Check sheet for the modelled part. Datum: model origin and axes. Units: mm. Face numbers are marked on the shaded views. A direction names the side the tool comes from. Coordinates: 2 decimals unless noted, no trailing zeros. Order: outer loops, then holes, each group sorted by start corner. A loop starts at its lowest first (then second) coordinate and runs counter-clockwise, first axis right, second up.
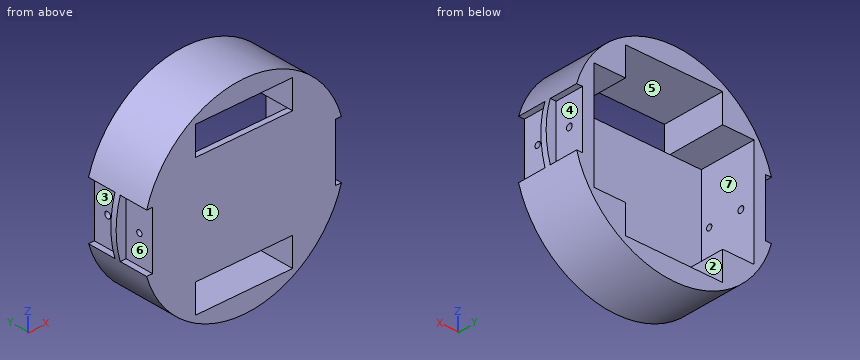
Autodesk Inventor part; units mm, degrees
ref_plane "YZ Plane" through (0, 0, 0) normal (1, 0, 0) x (0, 1, 0)
ref_plane "XZ Plane" through (0, 0, 0) normal (0, 1, 0) x (-1, 0, 0)
ref_plane "XY Plane" through (0, 0, 0) normal (0, 0, 1) x (1, 0, 0)
sketch "Szkic1" plane through (0, 0, 0) normal (0, 1, 0) x (-1, 0, 0)
  circle A0 centre (0, 0) radius 35.5
  line L0 (0, 18.75) -> (0, -18.75) construction
  line L1 (-28, 0) -> (28, 0) construction
  line L2 (-28, -18.75) -> (28, -18.75)
  line L3 (-28, 18.75) -> (-28, -18.75)
  line L4 (28, 18.75) -> (28, -18.75)
  line L5 (0, 18.75) -> (28, 18.75)
  line L6 (0, 18.75) -> (-28, 18.75)
  line L7 (0, 18.75) -> (0, 28.75) construction
  line L8 (17, 28.75) -> (-17, 28.75)
  line L9 (17, 28.75) -> (17, 18.75)
  line L10 (-17, 28.75) -> (-17, 18.75)
  line L11 (0, -18.75) -> (0, -28.75) construction
  line L12 (-17, -28.75) -> (17, -28.75)
  line L13 (17, -28.75) -> (17, -18.75)
  line L14 (-17, -28.75) -> (-17, -18.75)
  dimension "d0" = 71
  dimension "d1" = 37.5
  dimension "d2" = 56
  dimension "d4" = 10
  dimension "d5" = 34
  dimension "d16" = 10
  dimension "d17" = 34
extrude "Wyciągnięcie proste1" add sketch "Szkic1" along normal blind 20
extrude "Wyciągnięcie proste2" add sketch "Szkic1" against normal blind 2 contours A0 | L3 L6 L5 L4 L2
sketch "Szkic2" plane through (0, 20, 0) normal (0, 1, 0) x (1, 0, 0)
  line L0 (32, 0) -> (-32, 0) construction
  circle A0 centre (0, 0) radius 35.5
  line L1 (-32, -10) -> (-32, 10)
  line L2 (32, -10) -> (32, 10)
  line L3 (32, -10) -> (34.0624, -10)
  line L4 (32, 10) -> (34.0624, 10)
  line L5 (-32, -10) -> (-34.0624, -10)
  line L6 (-32, 10) -> (-34.0624, 10)
  dimension "d10" = 64
  dimension "d11" = 71
  dimension "d12" = 20
  dimension "d13" = 20
extrude "Wyciągnięcie proste3" cut sketch "Szkic2" against normal blind 10 contours A0 L3 L2 L4 | L6 L1 L5 A0
sketch "Szkic3" plane through (32, 20, 10) normal (1, 0, 0) x (0, 0, -1)
  line L0 (0, 0) -> (10, 0) construction
  line L1 (10, 0) -> (10, -5) construction
  circle A0 centre (10, -5) radius 1.1
  point P0 (10, -20)
  dimension "d18" = 10
  dimension "d19" = 20
  dimension "d20" = 20
  dimension "d21" = 5
  dimension "d22" = 2.2
extrude "Wyciągnięcie proste4" cut sketch "Szkic3" against normal through all
sketch "Szkic7" plane through (0, -2, 0) normal (0, -1, 0) x (1, 0, 0)
  line L0 (32, 0) -> (-32, 0) construction
  circle A0 centre (0, 0) radius 35.5
  line L1 (-32, -10) -> (-32, 10)
  line L2 (32, -10) -> (32, 10)
  line L3 (32, -10) -> (34.0624, -10)
  line L4 (32, 10) -> (34.0624, 10)
  line L5 (-32, -10) -> (-34.0624, -10)
  line L6 (-32, 10) -> (-34.0624, 10)
  dimension "d48" = 64
  dimension "d49" = 71
  dimension "d50" = 20
  dimension "d51" = 20
extrude "Wyciągnięcie proste8" cut sketch "Szkic7" against normal blind 10 contours A0 L3 L2 L4 | L6 L1 L5 A0
sketch "Szkic8" plane through (32, -2, 10) normal (1, 0, 0) x (0, 0, -1)
  line L0 (10, 2) -> (10, 5) construction
  circle A0 centre (10, 5) radius 1
  dimension "d54" = 3
  dimension "d55" = 2
extrude "Wyciągnięcie proste9" cut sketch "Szkic8" against normal through all
properties part number "002-002"
(1) Cross-section at A-A (x = 0). Enter the section's corners in (y, z).
Filled in:
outline: (-2, -35.5) - (20, -35.5) - (20, -28.75) - (-2, -28.75) - close; (-2, -18.75) - (0, -18.75) - (0, 18.75) - (-2, 18.75) - close; (-2, 28.75) - (20, 28.75) - (20, 35.5) - (-2, 35.5) - close
(2) Go/stop test with flat-tipped pins: P1, Ø2.5, axis at y = 3, z = 0, coming from the -X side; P2, Ø0.6, axis at x = -33, y = 15.5, coming from the +Z side; P3, Ø1, axis at y = 6.5, z = 13, coming from the +X side. Record where each tip stops, or that it passes through.
Filled in:
P1: stops at x = -32
P2: stops at z = 13.82
P3: stops at x = 33.23
(3) Cross-section at C-C (z = 0). Count the separate pieces of the cut face and the enclosed holes in it, and give its area (3 significant figures).
Filled in:
separate pieces: 5
enclosed holes: 0
area: 268 mm2
(4) Tool access check on the marked faces 4, 5, 6 and 7. Record the directions out of +Z, -Z, +X, -X, +Y, -Y that give a thin tool (end or side, any length) a straight path to the whole face; none if there is none.
Filled in:
face 4: +X, +Y
face 5: +Y, -Y
face 6: -X, -Y
face 7: +Y
(5) Thickness scan on probe 1 along Y at (x, z) = (29.05, 0); probe 2 along Z at (x, y) = (6, 11.5); probe 3 along Y at (x, z) = (-26, -10.5). Record the ranges inside material, lowest first.
Filled in:
probe 1: y = -2 to 2, 4 to 13.9, 16.1 to 20
probe 2: z = -34.99 to -28.75, 28.75 to 34.99
probe 3: y = -2 to 0
(6) Cross-section at D-D (y = 11). Enter the section's corners in (x, z), and give its area (3 significant figures).
Filled in:
outline: (-34.06, -10) arc R35.5 ccw to (34.06, -10) - (32, -10) - (32, 10) - (34.06, 10) arc R35.5 ccw to (-34.06, 10) - (-32, 10) - (-32, -10) - close; hole (-28, -18.75) - (-17, -18.75) - (-17, -28.75) - (17, -28.75) - (17, -18.75) - (28, -18.75) - (28, 18.75) - (17, 18.75) - (17, 28.75) - (-17, 28.75) - (-17, 18.75) - (-28, 18.75) - close
area: 1,060 mm2
(7) Cross-section at B-B (y = 15). Enter the section's corners in (x, z).
Filled in:
outline: (-34.06, -10) arc R35.5 ccw to (34.06, -10) - (32, -10) - (32, -1.1) - (28, -1.1) - (28, -18.75) - (17, -18.75) - (17, -28.75) - (-17, -28.75) - (-17, -18.75) - (-28, -18.75) - (-28, -1.1) - (-32, -1.1) - (-32, -10) - close; (-34.06, 10) - (-32, 10) - (-32, 1.1) - (-28, 1.1) - (-28, 18.75) - (-17, 18.75) - (-17, 28.75) - (17, 28.75) - (17, 18.75) - (28, 18.75) - (28, 1.1) - (32, 1.1) - (32, 10) - (34.06, 10) arc R35.5 ccw to start
(8) Release check for a two-part mould opening along X. For the marked faces 1, 2 and 3 record: +X half, -X half, draft (parallel to the pull), parting line (faces both ways), or undercut.
Filled in:
face 1: draft
face 2: undercut
face 3: -X half
